Input: part model. Units: mm. Frame: model coordinates. Round coordinates to 2 decimals unless told otherwise and drop trailing zeros. Order: outer loops, then holes, each group sorted by start corner. A loop starts at its lowest first (then second) coordinate and runs counter-clockwise, first axis right, second up.
Item 1: Cut plane C-C on x = 1.25. Output: boundary loops of the cut face in (y, z).
Item 2: Cut plane A-A on z = 23. Output: boundary loops of the cut face in (x, y), then the cut area to 3 significant figures.
Item 3: First-contact query: pin 1 (2.5 mm diameter, centred on x = 2.5, z = 14.5, fed in from +Y); pin 2 (0.7 mm diameter, centred on y = -0.5, z = 23, fed in from -X); pin 3 (3 mm diameter, centred on x = 2, z = 20, fed in from +Y). Flat tips, straight axial feed; report the tip coordinate or a pass-through.
Item 4: Cut plane D-D on z = 4.5. Output: boundary loops of the cut face in (x, y).
Item 5: Line query: L1, parallel to Y at x = -2.5, z = 19; L2, parallel to X at y = -0.25, z = 25.5. Output: solid intervals per line, ascending.
Item 6: Cut plane B-B on y = 2.5. Output: boundary loops of the cut face in (x, z), then the cut area to 3 significant figures.
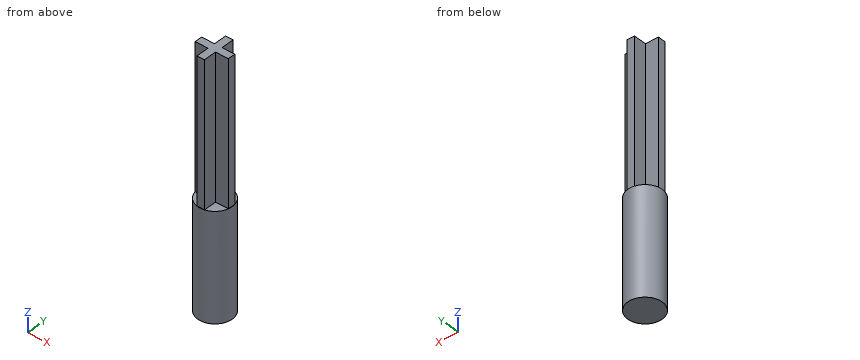
Autodesk Inventor part; units mm, degrees
ref_plane "YZ Plane" through (0, 0, 0) normal (1, 0, 0) x (0, 1, 0)
ref_plane "XZ Plane" through (0, 0, 0) normal (0, 1, 0) x (-1, 0, 0)
ref_plane "XY Plane" through (0, 0, 0) normal (0, 0, 1) x (1, 0, 0)
sketch "Sketch1" plane through (0, 0, 0) normal (0, 0, 1) x (1, 0, 0)
  circle A0 centre (0, 0) radius 3.048
  dimension "d0" = 6.096
extrude "Extrusion1" add sketch "Sketch1" along normal blind 38.1
sketch "Sketch2" plane through (0, 0, 0) normal (0, 0, -1) x (-1, 0, 0)
  circle A0 centre (0, 0) radius 3.048
extrude "Extrusion2" cut sketch "Sketch2" against normal blind 6.35
sketch "Sketch3" plane through (0, 0, 6.35) normal (0, 0, -1) x (-1, 0, 0)
  circle A0 centre (0, 0) radius 3.048
  line L0 (0, 0) -> (0, 0.6747) construction
  line L1 (-2.9727, 0.6731) -> (-0.6731, 0.6731)
  line L2 (0.6731, 0.6731) -> (2.9727, 0.6731)
  line L3 (-0.6731, 2.9727) -> (-0.6731, 0.6731)
  line L4 (-0.6731, -0.6731) -> (-0.6731, -2.9727)
  line L5 (0.6731, -2.9727) -> (0.6731, -0.6731)
  line L6 (0.6731, 0.6731) -> (0.6731, 2.9727)
  line L7 (-2.9727, -0.6731) -> (-0.6731, -0.6731)
  line L8 (0.6731, -0.6731) -> (2.9727, -0.6731)
  arc A1 (-0.6731, 2.9727) -> (-2.9727, 0.6731) centre (0, 0) ccw
  arc A2 (2.9727, 0.6731) -> (0.6731, 2.9727) centre (0, 0) ccw
  arc A3 (-2.9727, -0.6731) -> (-0.6731, -2.9727) centre (0, 0) ccw
  arc A4 (0.6731, -2.9727) -> (2.9727, -0.6731) centre (0, 0) ccw
  dimension "d5" = 1.3462
extrude "Extrusion3" cut sketch "Sketch3" against normal blind 31.75 contours L2 L6 A0 | A0 L5 L8 | L3 L1 A0 | A0 L7 L4
sketch "Sketch4" plane through (0, 0, 6.35) normal (0, 0, -1) x (-1, 0, 0)
  circle A0 centre (0, 0) radius 3.048
  line L0 (-0.6731, 2.9727) -> (0.6731, 2.9727)
  line L1 (-2.9727, -0.6731) -> (-2.9727, 0.6731)
  line L2 (0.6731, -2.9727) -> (-0.6731, -2.9727)
  line L3 (2.9727, 0.6731) -> (2.9727, -0.6731)
  arc A1 (0.6731, 2.9727) -> (-0.6731, 2.9727) centre (0, 0) ccw
  arc A2 (2.9727, -0.6731) -> (2.9727, 0.6731) centre (0, 0) ccw
  arc A3 (-2.9727, 0.6731) -> (-2.9727, -0.6731) centre (0, 0) ccw
  arc A4 (-0.6731, -2.9727) -> (0.6731, -2.9727) centre (0, 0) ccw
  point P0 (-0.6731, -2.9727)
  point P1 (2.9727, -0.6731)
  point P2 (-2.9727, 0.6731)
  dimension "d14" = 360
extrude "Extrusion4" cut sketch "Sketch4" against normal blind 25.4 contours A0 L3 | L0 A0 | A0 L2 | L1 A0
sketch "Sketch5" plane through (0, 0, 6.35) normal (0, 0, -1) x (-1, 0, 0)
  circle A0 centre (0, 0) radius 3.048
  dimension "d18" = 6.096
extrude "Extrusion5" add sketch "Sketch5" along normal blind 6.35
sketch "Sketch6" plane through (0, 0, 38.1) normal (0, 0, 1) x (1, 0, 0)
  circle A0 centre (0, 0) radius 3.048
  dimension "d21" = 6.096
extrude "Extrusion6" cut sketch "Sketch6" against normal blind 6.35
sketch "Sketch7" plane through (0, 0, 31.75) normal (0, 0, 1) x (1, 0, 0)
  line L0 (-0.6731, 2.9727) -> (0.6731, 2.9727)
  line L1 (0.6731, -0.6731) -> (0.6731, -2.9727)
  line L2 (-0.6731, 2.9727) -> (0.6731, 2.9727)
  line L3 (0.6731, -2.9727) -> (-0.6731, -2.9727)
  line L4 (-2.9727, -0.6731) -> (-2.9727, 0.6731)
  line L5 (2.9727, -0.6731) -> (2.9727, -0.6731)
  line L6 (2.9727, 0.6731) -> (2.9727, -0.6731)
  line L7 (-2.9727, -0.6731) -> (-2.9727, 0.6731)
  line L8 (-2.9727, 0.6731) -> (-0.6731, 0.6731)
  line L9 (0.6731, 0.6731) -> (2.9727, 0.6731)
  line L10 (-0.6731, -2.9727) -> (-0.6731, -0.6731)
  line L11 (-0.6731, 0.6731) -> (-0.6731, 2.9727)
  line L12 (0.6731, 2.9727) -> (0.6731, 0.6731)
  line L13 (0.6731, -0.6731) -> (0.6731, -2.9727)
  line L14 (2.9727, -0.6731) -> (0.6731, -0.6731)
  line L15 (-0.6731, -0.6731) -> (-2.9727, -0.6731)
  point P0 (0, 0)
sketch "Sketch8" plane through (0, 0, 0) normal (0, 0, -1) x (-1, 0, 0)
  circle A0 centre (0, 0) radius 3.048
extrude "Extrusion7" add sketch "Sketch8" along normal blind 12.7
properties part number "Bistable Rod"
From the geometry:
1. outline: (-2.78, -12.7) - (2.78, -12.7) - (2.78, 6.35) - (0.67, 6.35) - (0.67, 31.75) - (-0.67, 31.75) - (-0.67, 6.35) - (-2.78, 6.35) - close
2. outline: (-2.97, -0.67) - (-0.67, -0.67) - (-0.67, -2.97) - (0.67, -2.97) - (0.67, -0.67) - (2.97, -0.67) - (2.97, 0.67) - (0.67, 0.67) - (0.67, 2.97) - (-0.67, 2.97) - (-0.67, 0.67) - (-2.97, 0.67) - close
2. area: 14.2 mm2
3. pin 1: stops at y = 0.67
3. pin 2: stops at x = -2.97
3. pin 3: stops at y = 2.97
4. outline: circle Ø6.1 at (0, 0)
5. L1: y = -0.67 to 0.67
5. L2: x = -2.97 to 2.97
6. outline: (-1.74, -12.7) - (1.74, -12.7) - (1.74, 6.35) - (0.67, 6.35) - (0.67, 31.75) - (-0.67, 31.75) - (-0.67, 6.35) - (-1.74, 6.35) - close
6. area: 101 mm2
